Here's how the part is built. I have some questions about the finished solid (model axes, mm). A direction names the side the tool comes from. Round coordinates to 2 decimals unless told otherwise and drop trailing zeros. Write each loop counter-clockwise with the first axis right and the second up, starting at its lowest first coordinate (ties: lowest second). Pieces come first, ordered by that corner, then holes. Notation, with made-up numbers: M 20,-36 L 43,-36 A33 cw 43,-3 Z; hole C -33,60 d11. An arc over 180 degrees is marked long. Use a Markdown table: item, result. Add a question column.
```python
from build123d import *

# Parameters (mm, degrees)
SKETCH1_R           = 50
BOSS_EXTRUDE1_DEPTH = 35
SKETCH2_R           = 15
BOSS_EXTRUDE2_DEPTH = 270
SKETCH3_W           = 40
SKETCH3_H           = 40
BOSS_EXTRUDE3_DEPTH = 40


with BuildPart() as part:
    # Sketch1 → Boss-Extrude1 (new body)
    with BuildSketch(Plane(origin=(0, 0, 0), x_dir=(1, 0, 0), z_dir=(0, 1, 0))):
        Circle(SKETCH1_R)
    extrude(amount=BOSS_EXTRUDE1_DEPTH)

    # Sketch2 → Boss-Extrude2 (add)
    with BuildSketch(Plane(origin=(0, 35, 0), x_dir=(1, 0, 0), z_dir=(0, 1, 0))):
        Circle(SKETCH2_R)
    extrude(amount=BOSS_EXTRUDE2_DEPTH)

    # Sketch3 → Boss-Extrude3 (add)
    with BuildSketch(Plane(origin=(0, 305, 0), x_dir=(1, 0, 0), z_dir=(0, 1, 0))):
        Rectangle(SKETCH3_W, SKETCH3_H)
    extrude(amount=BOSS_EXTRUDE3_DEPTH)


solid = part.part
```
Item 1: For pin 1 Ø1.5 at (y, z) = (144.5, 9) entering from +X; pin 2 Ø5 at (x, y) = (9, 159) entering from +Z; pin 3 Ø4 at (x, z) = (3.5, 30) entering from +Y; pin 4 Ø1 at (x, z) = (-36, -36) entering from +Y, each with a flat end and sliding along its axis, tell me the tip position at first contact or that it passes through.
Item 2: Imagine slicing it at B-B on z = 3. List the corners of the cut face in (x, y) for me, plus the area to 3 significant figures.
Item 3: Imagine slicing it at A-A on x = 0. List the corners of the cut face in (y, z) for me.
Item 4: On a 3-axis mill with a long thin cutter (end or side, diameter ignored), from which of +Z, -Z, +X, -X, +Y, -Y can I reach the whole of each face in a straight line? I mean faces 5 (the face through (0, 345, 0)), 6 (the face through (-20, 325, 0)), 7 (the face through (0, 325, 20)), 8 (the face through (20, 325, 0)). Say none if no direction works.
Item 5: If we mould it in two halves opening along Y, with no side actions, what happens to faces 1 (the face through (9, 305, -14)), 2 (the face through (-14.985, 168.11, -0.66)), 3 (the face through (0, 325, -20)), 4 (the face through (-1, 0, -1))? For each: +Y half, -Y half, draft (parallel to the pull), parting line (faces both ways), or undercut.
Item 6: Imagine slicing it at C-C on y = 131.5. List the corners of the cut face in (x, z) for me, plus the area to 3 significant figures.
Item 7: I need wall thicknesses on probe 1 along Y at (x, z) = (-42, -16.5); probe 2 along Z at (x, y) = (0.5, 165.5); probe 3 along X at (y, z) = (118, -13). Which ranges of each line are inside material? Lowest first, please. Write a range as from..to.
Item 8: Imagine slicing it at D-D on z = 40. List the corners of the cut face in (x, y) for me, plus the area to 3 significant figures.
The answers:
| question | item | result |
|---|---|---|
| 1 | pin 1 | x = 12.53 |
| 1 | pin 2 | z = 13.52 |
| 1 | pin 3 | y = 35 |
| 1 | pin 4 | through |
| 2 | outline | M -49.91,0 L 49.91,0 L 49.91,35 L 14.7,35 L 14.7,305 L 20,305 L 20,345 L -20,345 L -20,305 L -14.7,305 L -14.7,35 L -49.91,35 Z |
| 2 | area | 13,000 mm² |
| 3 | outline | M 0,-50 L 35,-50 L 35,-15 L 305,-15 L 305,-20 L 345,-20 L 345,20 L 305,20 L 305,15 L 35,15 L 35,50 L 0,50 Z |
| 4 | face 5 | +Z, -Z, +X, -X, +Y |
| 4 | face 6 | +Z, -Z, -X, +Y |
| 4 | face 7 | +Z, +X, -X, +Y |
| 4 | face 8 | +Z, -Z, +X, +Y |
| 5 | face 1 | undercut |
| 5 | face 2 | undercut |
| 5 | face 3 | draft |
| 5 | face 4 | -Y half |
| 6 | outline | C 0,0 d30 |
| 6 | area | 707 mm² |
| 7 | probe 1 | 0..35 |
| 7 | probe 2 | -14.99..14.99 |
| 7 | probe 3 | -7.48..7.48 |
| 8 | outline | M -30,0 L 30,0 L 30,35 L -30,35 Z |
| 8 | area | 2,100 mm² |
